Here's how the part is built. I have some questions about the finished solid (model axes, mm). Face numbers are marked on the shaded views. A direction names the side the tool comes from. Round coordinates to 2 decimals unless told otherwise and drop trailing zeros. Loops run counter-clockwise (first coordinate to the right, second up) from the corner with the lowest first, then second, coordinate; pieces in that order, holes last. Notation, with made-up numbers: (64, 62.25) -> (87, 62.25) arc R21 cw to (87, 76.25) -> close; hole circle Ø5 at (-35, 4.5). An arc over 180 degrees is marked (long way). Use one line per item in the form item = value. Start each with the question number.
Item 1: If we section it at B-B (z = -34.5): Write out the boundary of the cut face in (x, y).
Item 2: If we section it at C-C (x = -5): Write out the boundary of the cut face in (y, z), then the cut area to 3 significant figures.
Item 3: If I drill on L1, parallel to Y at x = -5.5, z = -38; L2, parallel to Z at x = -6, y = 28; L3, parallel to X at y = 44.35, z = -34, over which ranges is the centre line in solid material (lowest first)? Write a range as [from, to].
Item 4: If we section it at A-A (y = 27): Write out the boundary of the cut face in (x, z), then the cut area to 3 significant figures.
Item 5: Thinking about a two-plate mould opening in Y: for the marked faces 1, 2 and 3, which applies, released by +Y, released by -Y, zero draft, split by the parting line, or undercut?
Item 6: I'm going to push flat-ended pins straight in: pin 1 Ø3.5 at (x, z) = (0, -33.47) entering from -Y; pin 2 Ø10 at (x, z) = (3.5, 16.5) entering from +Y (3 decimals); pin 3 Ø0.9 at (x, y) = (-2, 44.5) entering from -Z; pin 4 Ø1.5 at (x, y) = (1, 44) entering from +Z. Where does each tip first touch, or does it pass through?
Item 7: For the marked faces 4, 5 and 6, which set-ups out of +Z, -Z, +X, -X, +Y, -Y let a thin tool reach every point of the face, with its end or its side?
Item 8: If we section it at D-D (x = 0): State how many separate pieces and enclosed holes the cut face has, then the cut area to 3 significant figures.
```python
from build123d import *

# Parameters (mm, degrees)
SKETCH8_W          = 20
SKETCH8_H          = 3
SKETCH10_R         = 3
CUT_EXTRUDE1_DEPTH = 66.954529791
SKETCH11_R         = 3
CUT_EXTRUDE2_DEPTH = 66.954529791


with BuildPart() as part:
    # Sweep1: sweep along a path in Sketch7
    with BuildLine(Plane(origin=(0, 0, 0), x_dir=(0, 0, -1), z_dir=(1, 0, 0))) as sweep1_path:
        Line((-24, 46), (-44, 46))
        ThreePointArc((-44, 46), (-47.535533906, 44.535533906), (-49, 41))
        Line((-49, 41), (-49, 5))
        ThreePointArc((-49, 5), (-47.535533906, 1.464466094), (-44, 0))
        Line((-44, 0), (-23.473389189, 0))
        ThreePointArc((-23.473389189, 0), (-20.327624841, 1.113592061), (-18.583099774, 3.958333333))
        ThreePointArc((-18.583099774, 3.958333333), (0, 19), (18.583099774, 3.958333333))
        ThreePointArc((18.583099774, 3.958333333), (20.327624841, 1.113592061), (23.473389189, 0))
        Line((23.473389189, 0), (44, 0))
        ThreePointArc((44, 0), (47.535533906, 1.464466094), (49, 5))
        Line((49, 5), (49, 41))
        ThreePointArc((49, 41), (47.535533906, 44.535533906), (44, 46))
        Line((44, 46), (24, 46))
    # Sketch8 → Sweep1 (sweep)
    with BuildSketch(Plane.XY.offset(24)):
        with Locations((0, 44.5)):
            Rectangle(SKETCH8_W, SKETCH8_H)
    sweep(path=sweep1_path.line)

    # Sketch10 → Cut-Extrude1 (cut, through all)
    with BuildSketch(Plane(origin=(0, 3, 0), x_dir=(1, 0, 0), z_dir=(0, 1, 0))):
        with Locations(Location((0, 33.473389189, 0), (0, 0, 270))):
            Circle(SKETCH10_R)
        with Locations(Location((0, -33.473389189, 0), (0, 0, 270))):
            Circle(SKETCH10_R)
    extrude(amount=-CUT_EXTRUDE1_DEPTH, mode=Mode.SUBTRACT)

    # Sketch11 → Cut-Extrude2 (cut, through all)
    with BuildSketch(Plane.XZ.offset(-43)):
        with Locations(Location((0, 34, 0), (0, 0, 270))):
            Circle(SKETCH11_R)
        with Locations(Location((0, -34, 0), (0, 0, 270))):
            Circle(SKETCH11_R)
    extrude(amount=-CUT_EXTRUDE2_DEPTH, mode=Mode.SUBTRACT)


solid = part.part
```
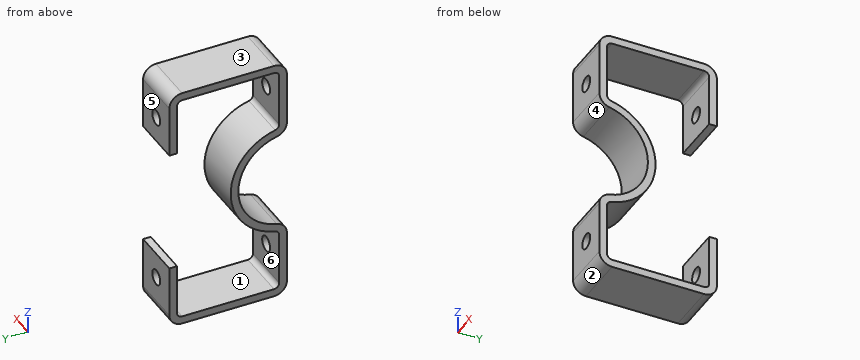
Values found:
q1.outline = (-10, 0) -> (-2.82, 0) -> (-2.82, 3) -> (-10, 3) -> close; (-10, 43) -> (-2.96, 43) -> (-2.96, 46) -> (-10, 46) -> close; (2.82, 0) -> (10, 0) -> (10, 3) -> (2.82, 3) -> close; (2.96, 43) -> (10, 43) -> (10, 46) -> (2.96, 46) -> close
q2.outline = (0, -44) arc R5 ccw to (5, -49) -> (41, -49) arc R5 ccw to (46, -44) -> (46, -24) -> (43, -24) -> (43, -44) arc R2 cw to (41, -46) -> (5, -46) arc R2 cw to (3, -44) -> (3, -23.47) arc R2 cw to (4.58, -21.52) arc R22 ccw to (4.58, 21.52) arc R2 cw to (3, 23.47) -> (3, 44) arc R2 cw to (5, 46) -> (41, 46) arc R2 cw to (43, 44) -> (43, 24) -> (46, 24) -> (46, 44) arc R5 ccw to (41, 49) -> (5, 49) arc R5 ccw to (0, 44) -> (0, 23.47) arc R5 ccw to (3.96, 18.58) arc R19 cw to (3.96, -18.58) arc R5 ccw to (0, -23.47) -> close
q2.area = 721 mm2
q3.L1 = [0, 3], [43, 46]
q3.L2 = [-49, -46], [46, 49]
q3.L3 = [-10, -3], [3, 10]
q4.outline = (-10, -49) -> (10, -49) -> (10, -46) -> (-10, -46) -> close; (-10, 46) -> (10, 46) -> (10, 49) -> (-10, 49) -> close
q4.area = 120 mm2
q5.face_1 = undercut
q5.face_2 = released by -Y
q5.face_3 = zero draft
q6.pin_1 = through
q6.pin_2 = 18.755
q6.pin_3 = -47.96
q6.pin_4 = 48.47
q7.face_4 = +X, -X, -Y
q7.face_5 = +Z, -Z, +X, -X, +Y
q7.face_6 = +X, -X
q8.separate_pieces = 5
q8.enclosed_holes = 0
q8.area = 649 mm2
